Geometry check sheet. Reference: the model listing, model coordinates, mm. Face numbers are marked on the shaded views. A direction names the side the tool comes from. Coordinates: 2 decimals unless noted, no trailing zeros. Write each loop counter-clockwise with the first axis right and the second up, starting at its lowest first coordinate (ties: lowest second). Pieces come first, ordered by that corner, then holes. Notation, with made-up numbers: (34.5, -23.5) -> (67.5, -23.5) arc R16 cw to (67.5, 3.5) -> close; hole circle Ø4 at (13.25, 26). An arc over 180 degrees is marked (long way). Answer in a Markdown table with one row per item. Add a question column.
1. Scan lines: L1, parallel to Z at x = 9.5, y = 0; L2, parallel to Y at x = 9.5, z = 12; L3, parallel to Y at x = 9, z = 12. Record each from-to range of solid material in increasing order. Write a range as from..to.
2. Depth check by flat-ended pin: P1, Ø8, axis at y = 15.5, z = 9.5, coming from the -X side; P2, Ø3, axis at x = 14, z = 9, coming from the -Y side; P3, Ø1.5, axis at x = 12.5, z = -7, coming from the +Y side; P4, Ø1, axis at y = 14, z = 16, coming from the +X side. Enter the tip coordinate at first touch or a pass-through.
3. Cross-section at A-A on x = 9.75. Record the cut outline in (y, z).
4. Cross-section at B-B on y = -9. Record the cut outline in (x, z).
5. Cross-section at D-D on z = 0. Record the cut outline in (x, y), and give its area (3 significant figures).
6. Set-up check for the marked faces 1, 2 and 3: record each of +Z, -Z, +X, -X, +Y, -Y from which the full face is reachable in a straight line by a thin tool's end or side.
7. Cross-section at C-C on y = 0. Record the cut outline in (x, z).
8. Mould release check, pull along Z, two halves, no side actions. Record for the marked faces 4, 5 and 6: pulls with the +Z half, pulls with the -Z half, needs draft (parallel to the pull), parting line crosses it, or undercut.
```python
from build123d import *

# Parameters (mm, degrees)
SKETCH1_R                               = 20
BLOCO_DEPTH                             = 22
ENCAIXE_START                           = -19
ENCAIXE_DO_POTENCI_METRO_DEPTH          = 19
FURO_DE_FIXA_O_PARAFUSO_M3_D            = 3.6
FURO_DE_FIXA_O_PARAFUSO_M3_CSINK_D      = 6.72
FURO_DE_FIXA_O_PARAFUSO_M3_CSINK_ANGLE  = 90
CORTE_ARREDONDAMENTO_DEPTH              = 36.832945734
CORTE_ARREDONDAMENTO_DEPTH_BACK         = 36.832945734
SKETCH7_R                               = 100
SKETCH7_R_2                             = 75
FURO_DE_FIXA_O_POTENCI_METRO_REACH      = 37.833
FURO_DE_FIXA_O_POTENCI_METRO_END_RADIUS = 20
SKETCH8_R                               = 1.5


with BuildPart() as part:
    # Sketch1 → Bloco (new body)
    with BuildSketch(Plane(origin=(0, 0, 0), x_dir=(0, 0, -1), z_dir=(1, 0, 0))):
        Circle(SKETCH1_R)
    extrude(amount=BLOCO_DEPTH)

    # Sketch2 → Encaixe do Potenciômetro (cut)
    with BuildSketch(Plane(origin=(22, 0, 0), x_dir=(0, 0, -1), z_dir=(1, 0, 0)).offset(ENCAIXE_START)):
        with BuildLine():
            Line((-8, -18.33030278), (-8, -2.015564437))
            ThreePointArc((-8, -2.015564437), (0, 8.25), (8, -2.015564437))
            Line((8, -2.015564437), (8, -18.33030278))
            ThreePointArc((8, -18.33030278), (0, -20), (-8, -18.33030278))
        make_face()
    extrude(amount=ENCAIXE_DO_POTENCI_METRO_DEPTH, mode=Mode.SUBTRACT)

    # Furo de Fixação - Parafuso M3 (through all)
    with Locations(Plane.ZY):
        with Locations((-12, 0), (12, 0)):
            CounterSinkHole(FURO_DE_FIXA_O_PARAFUSO_M3_D / 2, FURO_DE_FIXA_O_PARAFUSO_M3_CSINK_D / 2, counter_sink_angle=FURO_DE_FIXA_O_PARAFUSO_M3_CSINK_ANGLE)

    # Sketch7 → Corte - Arredondamento (cut, two sides: drawn at the far end of the back side and taken through both)
    with BuildSketch(Plane(origin=(0, 0, 0), x_dir=(1, 0, 0), z_dir=(0, 1, 0)).offset(-CORTE_ARREDONDAMENTO_DEPTH_BACK)):
        with Locations((75, 0)):
            Circle(SKETCH7_R)
        with Locations((75, 0)):
            Circle(SKETCH7_R_2, mode=Mode.SUBTRACT)
    extrude(amount=CORTE_ARREDONDAMENTO_DEPTH + CORTE_ARREDONDAMENTO_DEPTH_BACK, mode=Mode.SUBTRACT)

    # Furo de Fixação - Potenciômetro: up to this cylinder (the profile starts inside it)
    furo_de_fixa_o_potenci_metro_end = Plane(origin=(9.5, 0, 0), z_dir=(-1, 0, 0)) * Cylinder(FURO_DE_FIXA_O_POTENCI_METRO_END_RADIUS, 116.666, mode=Mode.PRIVATE)
    # Sketch8 → Furo de Fixação - Potenciômetro (cut, up to the surface)
    with BuildSketch(Plane.XY, mode=Mode.PRIVATE) as furo_de_fixa_o_potenci_metro_sk1:
        with Locations(Location((9.5, -9, 0), (0, 0, 180))):
            Circle(SKETCH8_R)
    furo_de_fixa_o_potenci_metro_tool1 = extrude(furo_de_fixa_o_potenci_metro_sk1.sketch, amount=FURO_DE_FIXA_O_POTENCI_METRO_REACH, mode=Mode.PRIVATE) & furo_de_fixa_o_potenci_metro_end
    add(furo_de_fixa_o_potenci_metro_tool1.solids().sort_by_distance((9.5, -9, 0))[0], mode=Mode.SUBTRACT)


solid = part.part
```
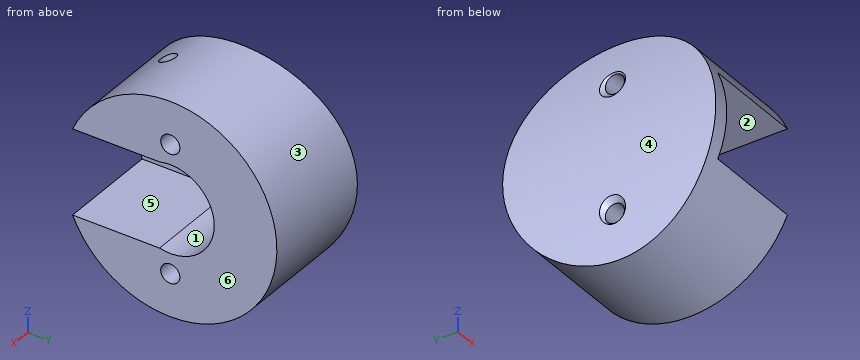
Results found:
| question | item | result |
|---|---|---|
| 1 | L1 | z = -20..-13.8, -10.2..-8.25, 8.25..10.2, 13.8..20 |
| 1 | L2 | y = -16..-10.5, -7.5..-1.8, 1.8..16 |
| 1 | L3 | y = -16..-10.41, -7.59..-1.8, 1.8..16 |
| 2 | P1 | stops at x = 0.2 |
| 2 | P2 | stops at y = -18.33 |
| 2 | P3 | stops at y = 19 |
| 2 | P4 | passes through |
| 3 | outline | (-18.33, -8) arc R20 ccw (long way) to (-7.52, 18.53) -> (-7.52, 8) -> (-2.02, 8) arc R8.25 cw (long way) to (-2.02, -8) -> close; (-18.33, 8) -> (-10.48, 8) -> (-10.48, 17.03) arc R20 ccw to start; hole circle Ø3.6 at (0, -12); hole circle Ø3.6 at (0, 12) |
| 4 | outline | (2.16, -17.86) -> (22, -17.86) -> (22, -8) -> (3, -8) -> (3, 8) -> (8, 8) -> (8, 17.86) -> (2.16, 17.86) arc R75 ccw to start; (11, 8) -> (22, 8) -> (22, 17.86) -> (11, 17.86) -> close |
| 5 | outline | (0, -20) -> (3, -20) -> (3, 8.25) -> (22, 8.25) -> (22, 20) -> (0, 20) -> close |
| 5 | area | 343 mm^2 |
| 6 | face 1 | +X |
| 6 | face 2 | +X, -Y |
| 6 | face 3 | +X, -X |
| 7 | outline | (0.57, -9.21) -> (1.56, -10.2) -> (22, -10.2) -> (22, -8.25) -> (3, -8.25) -> (3, 8.25) -> (22, 8.25) -> (22, 10.2) -> (1.56, 10.2) -> (0.57, 9.21) arc R75 ccw to start; (1.32, -14.04) arc R75 ccw to (2.72, -20) -> (22, -20) -> (22, -13.8) -> (1.56, -13.8) -> close; (1.32, 14.04) -> (1.56, 13.8) -> (22, 13.8) -> (22, 20) -> (2.72, 20) arc R75 ccw to start |
| 8 | face 4 | parting line crosses it |
| 8 | face 5 | undercut |
| 8 | face 6 | needs draft |
